from build123d import *

# Parameters (mm, degrees)
SKETCH1_R           = 1.65
BOSS_EXTRUDE1_DEPTH = 6
SKETCH2_R           = 3.5
BOSS_EXTRUDE2_DEPTH = 1
SKETCH4_R           = 1.65
CUT_EXTRUDE1_DEPTH  = 12
SKETCH7_R           = 9.5
CUT_EXTRUDE3_DEPTH  = 2
FILLET2_R           = 0.75
FILLET3_R           = 3.5
SKETCH8_R           = 3.15
SKETCH8_R_2         = 1.65
BOSS_EXTRUDE5_DEPTH = 0.4
CUT_EXTRUDE4_DEPTH  = 3


with BuildPart() as part:
    # Sketch1 → Boss-Extrude1 (new body)
    with BuildSketch(Plane.XY):
        with BuildLine():
            ThreePointArc((-0.145833333, -6.998480738), (7, 0), (-0.145833333, 6.998480738))
            Line((-0.145833333, 6.998480738), (-141.083984446, 4.06163185))
            ThreePointArc((-141.083984446, 4.06163185), (-149, 0), (-141.083984446, -4.06163185))
            Line((-141.083984446, -4.06163185), (-0.145833333, -6.998480738))
        make_face()
        with Locations((-144, 0)):
            Circle(SKETCH1_R, mode=Mode.SUBTRACT)
    extrude(amount=BOSS_EXTRUDE1_DEPTH)

    # Sketch2 → Boss-Extrude2 (add)
    with BuildSketch(Plane.XY.offset(6)):
        Circle(SKETCH2_R)
    extrude(amount=BOSS_EXTRUDE2_DEPTH)

    # Sketch4 → Cut-Extrude1 (cut)
    with BuildSketch(Plane.XY.offset(7)):
        Circle(SKETCH4_R)
    extrude(amount=-CUT_EXTRUDE1_DEPTH, mode=Mode.SUBTRACT)

    # Sketch7 → Cut-Extrude3 (cut)
    with BuildSketch(Plane.XY.offset(6)):
        with Locations((-144, 0)):
            Circle(SKETCH7_R)
    extrude(amount=-CUT_EXTRUDE3_DEPTH, mode=Mode.SUBTRACT)

    # Fillet2
    fillet2_edges = [part.edges().sort_by_distance(p)[0] for p in [
        (-135.468359541, 4.178649433, 5),
        (-135.468359541, -4.178649433, 5),
    ]]
    fillet(fillet2_edges, radius=FILLET2_R)

    # Fillet3
    fillet3_edges = [part.edges().sort_by_distance(p)[0] for p in [
        (-141.083984446, -4.06163185, 2),
        (-141.083984446, 4.06163185, 2),
    ]]
    fillet(fillet3_edges, radius=FILLET3_R)

    # Sketch8 → Boss-Extrude5 (add)
    with BuildSketch(Plane.XY.offset(4)):
        with Locations((-144, 0)):
            Circle(SKETCH8_R)
        with Locations((-144, 0)):
            Circle(SKETCH8_R_2, mode=Mode.SUBTRACT)
    extrude(amount=BOSS_EXTRUDE5_DEPTH)

    # Sketch9 → Cut-Extrude4 (cut)
    with BuildSketch(Plane.XY.offset(6)):
        with BuildLine():
            Line((-8.018864585, -3.833772393), (-106.262176435, -1.786592415))
            ThreePointArc((-106.262176435, -1.786592415), (-107.476577581, -1.260839283), (-107.975717263, -0.035259389))
            ThreePointArc((-107.975717263, -0.035259389), (-107.975700008, 0), (-107.975717263, 0.035259389))
            ThreePointArc((-107.975717263, 0.035259389), (-107.476577581, 1.260839283), (-106.262176435, 1.786592415))
            Line((-106.262176435, 1.786592415), (-8.018864585, 3.833772393))
            ThreePointArc((-8.018864585, 3.833772393), (-6.60867738, 3.168296566), (-6.289168562, 1.642059316))
            ThreePointArc((-6.289168562, 1.642059316), (-6.5, 0), (-6.289168562, -1.642059316))
            ThreePointArc((-6.289168562, -1.642059316), (-6.60867738, -3.168296566), (-8.018864585, -3.833772393))
        make_face()
    extrude(amount=-CUT_EXTRUDE4_DEPTH, mode=Mode.SUBTRACT)


solid = part.part
Read the model definition and answer for the solid it produces. Units are mm, in the model's axes. A direction names the side the tool comes from. Round coordinates to 2 decimals unless told otherwise and drop trailing zeros. Order: outer loops, then holes, each group sorted by start corner. A loop starts at its lowest first (then second) coordinate and runs counter-clockwise, first axis right, second up.
1) The part is cut by section C-C on x = -48. Write down the section's boundary in (y, z), plus the area to 3 significant figures.
2) For faces 1 (the face through (-142.6, -1.4, 4.4)), 2 (the face through (-6.5, 0, 4.5)), 3 (the face through (1, -2, 7)), determine the directions among +Z, -Z, +X, -X, +Y, -Y from which every point of the face is accessible in a straight line to the end or side of a thin tool.
3) Straight lines are drawn through the part: L1, parallel to Y at x = 0, z = 2; L2, parallel to Y at x = -144, z = 1.7; L3, parallel to Z at x = -126.5, y = -3.75. For each, find the intervals that lie inside material, in ascending order.
4) The part is cut by section A-A on x = -144. Write down the section's boundary in (y, z), plus the area to 3 significant figures.
5) The part is cut by section B-B on x = -25.5. Write down the section's boundary in (y, z), plus the area to 3 significant figures.
6) Flat-ended cylindrical pins translate along their axes: pin 1 (4 mm diameter, centred on x = 0, y = 0, fed in from +Z); pin 2 (4 mm diameter, centred on x = -60.5, y = -2, fed in from +Z); pin 3 (8 mm diameter, centred on x = -141, y = -0.5, fed in from +Z); pin 4 (2.5 mm diameter, centred on x = -68, y = -0.5, fed in from +Z). Find the tip coordinate at first contact, or state that the pin passes through.
7) The mould has two halves that part along Y. Classify faces 4 (the face through (-72, 0, 0)), 5 (the face through (-45, 0, 3)), 6 (the face through (-149, 0, 2)), 7 (the face through (-142.426, 0.496, 2.169)): released by +Y, released by -Y, zero draft, split by the parting line, or undercut.
Resolved:
1. outline: (-6, 0) - (6, 0) - (6, 6) - (3, 6) - (3, 3) - (-3, 3) - (-3, 6) - (-6, 6) - close
1. area: 54.0 mm2
2. face 1: +Z, -X, +Y, -Y
2. face 2: +Z
2. face 3: +Z, +X, -X, +Y, -Y
3. L1: y = -7 to -1.65, 1.65 to 7
3. L2: y = -5 to -1.65, 1.65 to 5
3. L3: z = 0 to 6
4. outline: (-5, 0) - (-1.65, 0) - (-1.65, 4.4) - (-3.15, 4.4) - (-3.15, 4) - (-5, 4) - close; (1.65, 0) - (5, 0) - (5, 4) - (3.15, 4) - (3.15, 4.4) - (1.65, 4.4) - close
4. area: 28.0 mm2
5. outline: (-6.47, 0) - (6.47, 0) - (6.47, 6) - (3.47, 6) - (3.47, 3) - (-3.47, 3) - (-3.47, 6) - (-6.47, 6) - close
5. area: 56.8 mm2
6. pin 1: stops at z = 7
6. pin 2: stops at z = 6
6. pin 3: stops at z = 4.4
6. pin 4: stops at z = 3
7. face 4: zero draft
7. face 5: undercut
7. face 6: split by the parting line
7. face 7: undercut
